Input: part model. Units: mm. Frame: model coordinates. A direction names the side the tool comes from. Round coordinates to 2 decimals unless told otherwise and drop trailing zeros. Loops run counter-clockwise (first coordinate to the right, second up) from the corner with the lowest first, then second, coordinate; pieces in that order, holes last. Notation, with made-up numbers: (-12.75, -28) - (23.25, -28) arc R22 ccw to (23.25, 3) - close; hole circle Ø8 at (4.5, 88). An arc over 180 degrees is marked (long way). One line per question, with ' | ' between items. Start each with the question number.
Item 1: Section C-C, the plane y = 26. Return loops of the section in (x, z).
Item 2: First-contact query: pin 1 (1.1 mm diameter, centred on x = -43.5, z = 15.5, fed in from +Y); pin 2 (1.8 mm diameter, centred on y = -2.5, z = 14, fed in from -X); pin 3 (3 mm diameter, centred on y = 44, z = 15.5, fed in from +X). Flat tips, straight axial feed; report the tip coordinate or a pass-through.
Item 3: Section A-A, the plane x = -17. Return loops of the section in (y, z).
Item 4: Section B-B, the plane z = 11.25. Return loops of the section in (x, y).
Item 5: Draft query along Z for faces 1 (the face through (-32.09, 20.24, 14.3)), 2 (the face through (-20.24, 9.77, 14.3)), 3 (the face through (-27, 27, 10)), 4 (the face through (-37.93, 44, 14)). Return one class per face: pulls with the +Z half, pulls with the -Z half, needs draft (parallel to the pull), parting line crosses it, or undercut.
Item 6: Section D-D, the plane x = -2.5. Return loops of the section in (y, z), plus the area to 3 significant figures.
Item 7: Material intervals for line 1 along X through (y, z) = (10, 14); line 2 along Y through (x, z) = (-33, 14); line 3 along Y through (x, z) = (-42.75, 14), sorted ascending.
Item 8: Set-up query: faces 5 (the face through (-3.971, -2, 14)), 6 (the face through (-44, 3.93, 14)), 7 (the face through (-3.93, 44, 14)), 8 (the face through (-35.83, 20, 14)), 9 (the face through (-22.657, 1.1, 10.662)). Return all of +Z, -Z, +X, -X, +Y, -Y with unobstructed straight access to the full face (end or side cutting, diameter ignored); none if empty.
Autodesk Inventor part; units mm, degrees
ref_plane "Work Plane1" through (0, 0, 10) normal (0, 0, 1) x (1, 0, 0)
ref_plane "YZ Plane" through (0, 0, 0) normal (1, 0, 0) x (0, 1, 0)
ref_plane "XZ Plane" through (0, 0, 0) normal (0, 1, 0) x (-1, 0, 0)
ref_plane "Work Plane1" through (0, 0, 10) normal (0, 0, 1) x (1, 0, 0)
sketch "Sketch1" plane through (0, 0, 10) normal (0, 0, 1) x (1, 0, 0)
  line L0 (-4.0299, -0.3538) -> (-2.2322, 1.4439) construction
  arc A0 (-1.4439, 2.2322) -> (-2.2322, 1.4439) centre (-0.9299, 0.9299) ccw construction
  line L1 (-1.4439, 2.2322) -> (0.3538, 4.0299) construction
  line L2 (-37.8299, 42.8299) -> (-37.8299, 37.8299) construction
  line L3 (-37.8299, 37.8299) -> (-42.9208, 37.8299) construction
  line L4 (-37.8299, 42.2137) -> (-37.8299, 45.8299) construction
  line L5 (-37.8299, 45.8299) -> (-4.0299, 45.8299) construction
  line L6 (-4.0299, 45.8299) -> (-4.0299, 42.2137) construction
  line L7 (-4.0299, 4.0299) -> (0.3538, 4.0299)
  circle A1 centre (-20.9299, 20.9299) radius 17.5
  line L8 (-20.9299, 58.9723) -> (17.1124, 20.9299) construction
  line L9 (17.1124, 20.9299) -> (-20.9299, -17.1124) construction
  line L10 (-20.9299, -17.1124) -> (-58.9723, 20.9299) construction
  line L11 (-58.9723, 20.9299) -> (-20.9299, 58.9723) construction
  line L12 (-20.9299, 58.9723) -> (-20.9299, -17.1124) construction
  line L13 (17.1124, 20.9299) -> (-58.9723, 20.9299) construction
  line L14 (-20.9299, 58.9723) -> (32.8701, 58.9723) construction
  line L15 (-43.4299, 43.4299) -> (1.5701, 43.4299) construction
  line L16 (1.5701, 43.4299) -> (1.5701, -1.5701) construction
  line L17 (1.5701, -1.5701) -> (-43.4299, -1.5701) construction
  line L18 (-43.4299, -1.5701) -> (-43.4299, 43.4299) construction
  line L19 (-43.4299, 43.4299) -> (1.5701, -1.5701) construction
  line L20 (1.5701, 43.4299) -> (-43.4299, -1.5701) construction
  line L21 (-43.4299, 5.3876) -> (-43.4299, 36.4723)
  line L22 (-43.4299, 36.4723) -> (-36.4723, 43.4299)
  line L23 (-36.4723, 43.4299) -> (-5.3876, 43.4299)
  line L24 (-5.3876, 43.4299) -> (1.5701, 36.4723)
  line L25 (1.5701, 36.4723) -> (1.5701, 5.3876)
  line L26 (1.5701, 5.3876) -> (-5.3876, -1.5701)
  line L27 (-5.3876, -1.5701) -> (-36.4723, -1.5701)
  line L28 (-36.4723, -1.5701) -> (-43.4299, 5.3876)
  line L29 (-4.0299, 42.2137) -> (-37.8299, 42.2137)
  line L30 (-4.0299, -0.3538) -> (-4.0299, 4.0299)
  circle A2 centre (-20.9299, 20.9299) radius 1.5
  line L31 (-10.9299, 10.9299) -> (-30.9299, 10.9299) construction
  line L32 (-30.9299, 10.9299) -> (-30.9299, 30.9299) construction
  line L33 (-30.9299, 30.9299) -> (-10.9299, 30.9299) construction
  line L34 (-10.9299, 30.9299) -> (-10.9299, 10.9299) construction
  line L35 (-10.9299, 10.9299) -> (-30.9299, 30.9299) construction
  line L36 (-30.9299, 10.9299) -> (-10.9299, 30.9299) construction
  circle A3 centre (-30.9299, 30.9299) radius 1.4
  circle A4 centre (-30.9299, 10.9299) radius 1.4
  circle A5 centre (-10.9299, 10.9299) radius 1.4
  line L37 (-45.8299, 37.8299) -> (-42.0723, 37.8299) construction
  line L38 (-42.1723, 37.7299) -> (-45.8299, 37.7299)
  line L39 (-45.8299, 37.7299) -> (-45.8299, 4.1299)
  line L40 (-45.8299, 4.1299) -> (-42.1723, 4.1299)
  line L41 (-42.1723, 4.1299) -> (-42.1723, 37.7299)
  line L42 (-45.8299, 4.0299) -> (-42.0723, 4.0299) construction
  line L43 (-45.8299, 37.8299) -> (-42.0723, 37.8299)
  line L44 (-37.7299, 45.8299) -> (-4.1299, 45.8299)
  line L45 (-4.1299, 45.8299) -> (-4.1299, 42.1723)
  line L46 (-4.1299, 42.1723) -> (-37.7299, 42.1723)
  line L47 (-37.7299, 42.1723) -> (-37.7299, 45.8299)
  line L48 (0.4701, 37.8299) -> (0.4701, 4.0299) construction
  line L49 (0.4701, 4.0299) -> (3.9701, 4.0299) construction
  line L50 (3.9701, 37.8299) -> (3.9701, 4.0299) construction
  line L51 (0.4701, 37.8299) -> (3.9701, 37.8299) construction
  line L52 (-45.8299, -3.9701) -> (-4.0299, -3.9701) construction
  line L53 (0.3124, 37.7299) -> (3.9701, 37.7299)
  line L54 (3.9701, 37.7299) -> (3.9701, 4.1299)
  line L55 (3.9701, 4.1299) -> (0.3124, 4.1299)
  line L56 (0.3124, 4.1299) -> (0.3124, 37.7299)
  line L57 (-4.1713, -0.3538) -> (-37.7299, -0.3538)
  line L58 (-37.7299, -0.3538) -> (-37.7299, -3.9701)
  line L59 (-37.7299, -3.9701) -> (-4.1713, -3.9701)
  line L60 (-4.1713, -3.9701) -> (-4.1713, -0.3538)
  point P0 (-37.8299, 4.0299)
  dimension "d18" = 53.8
  dimension "d19" = 45
  dimension "d20" = 53.8
  dimension "d21" = 45
  dimension "d22" = 45
  dimension "d30" = 20
  dimension "d31" = 20
  dimension "d32" = 2.8
  dimension "d33" = 2.8
  dimension "d34" = 2.8
  dimension "d35" = 3
  dimension "d36" = 0.1
  dimension "d37" = 0.1
  dimension "d38" = 0.1
  dimension "d39" = 0.1
extrude "Extrusion1" add sketch "Sketch1" along normal blind 8 contours L30 L26 L57 L28 L41 L22 L46 L24 L56 L7 | L7 L26 L30 | L56 L24 L25 L26 | L26 L25 L24 L53 L54 L55 | L60 L59 L58 L57 L28 L27 L26 | L26 L27 L28 L57 | L46 L22 L29 L24 | L24 L29 L45 | L40 L39 L38 L22 L21 L28 | L28 L21 L22 L41 | L29 L22 L23 L24 | L24 L23 L22 L29 L47 L44 L45 | L47 L29 L22 | A1 | A2 | A3 | A4 | A5
sketch "Skizze4" plane through (0, 0, 18) normal (0, 0, 1) x (1, 0, 0)
  line L0 (-37.7299, 42.1723) -> (-42.1723, 37.7299)
  line L1 (-42.1723, 37.7299) -> (-45.8299, 37.7299)
  line L2 (-45.8299, 37.7299) -> (-45.8299, 4.1299) construction
  line L3 (-45.8299, 4.1299) -> (-42.1723, 4.1299)
  line L4 (-42.1723, 4.1299) -> (-37.6885, -0.3538)
  line L5 (-37.6885, -0.3538) -> (-37.7299, -0.3538)
  line L6 (-37.7299, -0.3538) -> (-37.7299, -3.9701)
  line L7 (-37.7299, -3.9701) -> (-4.1713, -3.9701) construction
  line L8 (-4.1713, -3.9701) -> (-4.1713, -0.3538)
  line L9 (-4.1713, -0.3538) -> (0.3124, 4.1299)
  line L10 (0.3124, 4.1299) -> (3.9701, 4.1299)
  line L11 (3.9701, 4.1299) -> (3.9701, 37.7299) construction
  line L12 (3.9701, 37.7299) -> (0.3124, 37.7299)
  line L13 (0.3124, 37.7299) -> (-4.1299, 42.1723)
  line L14 (-4.1299, 42.1723) -> (-4.1299, 45.8299)
  line L15 (-4.1299, 45.8299) -> (-37.7299, 45.8299) construction
  line L16 (-37.7299, 45.8299) -> (-37.7299, 42.1723)
  line L17 (-37.9299, 46.0299) -> (-3.9299, 46.0299) construction
  line L18 (-3.9299, 46.0299) -> (-3.9299, 42.2551)
  line L19 (-3.9299, 42.2551) -> (0.3953, 37.9299)
  line L20 (0.3953, 37.9299) -> (4.1701, 37.9299)
  line L21 (4.1701, 37.9299) -> (4.1701, 3.9299) construction
  line L22 (4.1701, 3.9299) -> (0.3953, 3.9299)
  line L23 (0.3953, 3.9299) -> (-3.9713, -0.4367)
  line L24 (-3.9713, -0.4367) -> (-3.9713, -4.1701)
  line L25 (-3.9713, -4.1701) -> (-37.9299, -4.1701) construction
  line L26 (-37.9299, -4.1701) -> (-37.9299, -0.3953)
  line L27 (-37.9299, -0.3953) -> (-42.2551, 3.9299)
  line L28 (-42.2551, 3.9299) -> (-46.0299, 3.9299)
  line L29 (-46.0299, 3.9299) -> (-46.0299, 37.9299) construction
  line L30 (-46.0299, 37.9299) -> (-42.2551, 37.9299)
  line L31 (-42.2551, 37.9299) -> (-37.9299, 42.2551)
  line L32 (-37.9299, 42.2551) -> (-37.9299, 46.0299)
  line L33 (-45.8299, 37.7299) -> (-45.8299, 37.9299)
  line L34 (-4.1299, 45.8299) -> (-37.7299, 45.8299)
  line L35 (-37.7299, 45.8299) -> (-37.9299, 45.8299)
  line L36 (-4.1299, 45.8299) -> (-3.9299, 45.8299)
  line L37 (3.9701, 37.7299) -> (3.9701, 37.9299)
  line L38 (3.9701, 4.1299) -> (3.9701, 37.7299)
  line L39 (3.9701, 4.1299) -> (3.9701, 3.9299)
  line L40 (-4.1713, -3.9701) -> (-3.9713, -3.9701)
  line L41 (-37.7299, -3.9701) -> (-37.9299, -3.9701)
  line L42 (-45.8299, 4.1299) -> (-45.8299, 3.9299)
  point P0 (0, 0)
  dimension "d40" = 0.2
extrude "IM_offset" add sketch "Skizze4" against normal up to surface (8 mm away)
sketch "Sketch25" plane through (0, 0, 10) normal (0, 0, -1) x (-1, 0, 0)
  circle A0 centre (20.9299, 20.9299) radius 7.8
  line L0 (3.9713, -3.9701) -> (37.9299, -3.9701)
  line L1 (37.9299, -3.9701) -> (37.9299, -0.3953)
  line L2 (37.9299, -0.3953) -> (42.2551, 3.9299)
  line L3 (42.2551, 3.9299) -> (45.8299, 3.9299)
  line L4 (45.8299, 3.9299) -> (45.8299, 37.9299)
  line L5 (45.8299, 37.9299) -> (42.2551, 37.9299)
  line L6 (42.2551, 37.9299) -> (37.9299, 42.2551)
  line L7 (37.9299, 42.2551) -> (37.9299, 45.8299)
  line L8 (37.9299, 45.8299) -> (3.9299, 45.8299)
  line L9 (3.9299, 45.8299) -> (3.9299, 42.2551)
  line L10 (3.9299, 42.2551) -> (-0.3953, 37.9299)
  line L11 (-0.3953, 37.9299) -> (-3.9701, 37.9299)
  line L12 (-3.9701, 37.9299) -> (-3.9701, 3.9299)
  line L13 (-3.9701, 3.9299) -> (-0.3953, 3.9299)
  line L14 (-0.3953, 3.9299) -> (3.9713, -0.4367)
  line L15 (3.9713, -0.4367) -> (3.9713, -3.9701)
  circle A1 centre (20.9299, 20.9299) radius 24.9
  point P0 (0, 0)
  dimension "d167" = 15.6
extrude "Extrusion21" cut sketch "Sketch25" against normal through all contours A0
sketch "Sketch26" plane through (-37.9299, -3.9701, 10) normal (0, -1, 0) x (1, 0, 0)
  line L0 (8.25, 4.8) -> (8.25, 11.5)
  line L1 (10.75, 4.8) -> (10.75, 11.5)
  circle A0 centre (16.3239, 4) radius 1.4
  line L2 (33.9586, 8) -> (0, 8)
  point P0 (37.9299, -10)
  dimension "d155" = 2.8
  dimension "d156" = 4
hole "Hole1" at (-21.606, -3.9701, 14) direction (0, 1, 0) diameter 2.8 end through all counterbore diameter 7 counterbore depth 10
pattern_circular "Circular Pattern1" count 2 over 90 about axis through (-20.9299, 20.9299, 10) along (0, 0, -1) of "Hole1", "Extrusion21"
properties part number "20_Cube_Insert_Fiber_STMount_Center"
Return value:
1) outline: (-45.83, 10) - (-26.86, 10) - (-26.86, 18) - (-45.83, 18) - close; (-15, 10) - (3.97, 10) - (3.97, 18) - (-15, 18) - close
2) pin 1: y = 37.93 | pin 2: x = -37.93 | pin 3: x = -3.93
3) outline: (-3.97, 10) - (14.19, 10) - (14.19, 18) - (-3.97, 18) - close; (27.67, 10) - (45.83, 10) - (45.83, 18) - (27.67, 18) - close
4) outline: (-45.83, 3.93) - (-42.26, 3.93) - (-37.93, -0.4) - (-37.93, -3.97) - (-23.77, -3.97) - (-23.77, 6.03) - (-19.44, 6.03) - (-19.44, -3.97) - (-3.97, -3.97) - (-3.97, -0.44) - (0.4, 3.93) - (3.97, 3.93) - (3.97, 37.93) - (0.4, 37.93) - (-3.93, 42.26) - (-3.93, 45.83) - (-37.93, 45.83) - (-37.93, 42.26) - (-42.26, 37.93) - (-45.83, 37.93) - (-45.83, 23.77) - (-35.83, 23.77) - (-35.83, 19.44) - (-45.83, 19.44) - close; hole circle Ø15.6 at (-20.93, 20.93)
5) face 1: undercut | face 2: undercut | face 3: pulls with the -Z half | face 4: needs draft
6) outline: (1.03, 10) - (40.83, 10) - (40.83, 18) - (1.03, 18) - close; hole circle Ø2.8 at (21.61, 14) | area: 312 mm2
7) line 1: -45.83 to -23.01, -20.21 to 3.97 | line 2: -3.97 to 20.21, 23.01 to 45.83 | line 3: 3.93 to 18.11, 25.11 to 37.93
8) face 5: +Z, -Z, +X, -Y | face 6: +Z, -Z, -X, -Y | face 7: +Z, -Z, +X, +Y | face 8: -X | face 9: -Y
